from build123d import *

# Parameters (mm, degrees)
F0_W     = 140
F0_H     = 160
F0_W_2   = 100
F0_H_2   = 120
F1_DEPTH = 2
F2_DEPTH = 5
F3_DEPTH = 10


with BuildPart() as f1:
    # F0 (on Top) → F1 (new body)
    with BuildSketch(Plane.XY):
        with Locations((50, 60)):
            Rectangle(F0_W, F0_H)
        with Locations((50, 60)):
            Rectangle(F0_W_2, F0_H_2, mode=Mode.SUBTRACT)
        with Locations((50, 60)):
            Rectangle(F0_W_2, F0_H_2)
    extrude(amount=F1_DEPTH)

    # F0 (on Top) → F2 (join)
    with BuildSketch(Plane.XY):
        with Locations((50, 60)):
            Rectangle(F0_W_2, F0_H_2)
    extrude(amount=F2_DEPTH)

    # F0 (on Top) → F3 (join)
    with BuildSketch(Plane.XY):
        with Locations((50, 60)):
            Rectangle(F0_W, F0_H)
        with Locations((50, 60)):
            Rectangle(F0_W_2, F0_H_2, mode=Mode.SUBTRACT)
        with Locations((50, 60)):
            Rectangle(F0_W_2, F0_H_2)
    extrude(amount=-F3_DEPTH)


solid = f1.part
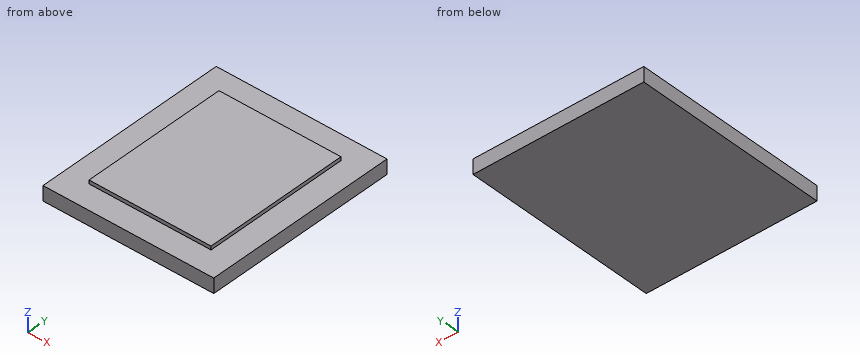
Work out the finished part from the listing and answer in its coordinate system (mm). Give positions to 0.01 mm unless a question says otherwise; leave off trailing zeros. Order: outer loops, then holes, each group sorted by start corner. A loop starts at its lowest first (then second) coordinate and runs counter-clockwise, first axis right, second up. Notation, with made-up numbers: (12, -15.75) -> (59, -15.75) arc R16 ccw to (59, -4.75) -> close; hole circle Ø8 at (-16.5, 2). An arc over 180 degrees is marked (long way). Answer as a JSON object with one key per item and string values. Group by question number.
1. Section B-B on x = 89 is taken. Determine the outline of the cut face in (y, z).
2. Section C-C on y = 123 is taken. Determine the outline of the cut face in (x, z).
3. Flat-ended cylindrical pins translate along their axes: pin 1 Ø2.5 at (x, z) = (45, 4) entering from -Y; pin 2 Ø1.5 at (y, z) = (62, 4) entering from -X; pin 3 Ø0.9 at (x, z) = (26.5, 3.5) entering from +Y. Find the tip coordinate at first contact, or state that the pin passes through.
4. Section A-A on y = 89.5 is taken. Determine the outline of the cut face in (x, z), plus the area to 3 significant figures.
5. Consider line 1 along Y through (x, z) = (55.5, 2.5); line 2 along Z through (x, y) = (77, 127.5); line 3 along X through (y, z) = (60.5, 3.25). Determine where each line is inside the solid, lowest interval first. Write a range as [from, to].
Result sheet:
{
 "1": {"outline": "(-20, -10) -> (140, -10) -> (140, 2) -> (120, 2) -> (120, 5) -> (0, 5) -> (0, 2) -> (-20, 2) -> close"},
 "2": {"outline": "(-20, -10) -> (120, -10) -> (120, 2) -> (-20, 2) -> close"},
 "3": {"pin 1": "stops at y = 0", "pin 2": "stops at x = 0", "pin 3": "stops at y = 120"},
 "4": {"outline": "(-20, -10) -> (120, -10) -> (120, 2) -> (100, 2) -> (100, 5) -> (0, 5) -> (0, 2) -> (-20, 2) -> close", "area": "1,980 mm^2"},
 "5": {"line 1": "y = [0, 120]", "line 2": "z = [-10, 2]", "line 3": "x = [0, 100]"}
}
